Verification items for the finished model (mm, model axes). Give positions to 0.01 mm unless a question says otherwise; leave off trailing zeros. Order: outer loops, then holes, each group sorted by start corner. A loop starts at its lowest first (then second) coordinate and runs counter-clockwise, first axis right, second up.
from build123d import *

# Parameters (mm, degrees)
SKETCH1_R                           = 14.2875
BOSS_EXTRUDE1_DEPTH                 = 6.35
F_0_257_DIAMETER_HOLE1_D            = 6.5278
F_9_0_2_DIAMETER_HOLE1_D            = 5.08
FILLET2_R                           = 12.7
FILLET1_R                           = 19.05
F_9_0_196_DIAMETER_HOLE1_AT_2_COUNT = 2
F_9_0_196_DIAMETER_HOLE1_AT_2_PITCH = 25.4
F_9_0_196_DIAMETER_HOLE1_AT_3_COUNT = 2
F_9_0_196_DIAMETER_HOLE1_AT_3_PITCH = 76.2
F_9_0_196_DIAMETER_HOLE1_AT_4_COUNT = 2
F_9_0_196_DIAMETER_HOLE1_AT_4_PITCH = 101.6


with BuildPart() as part:
    # Sketch1 → Boss-Extrude1 (new body)
    with BuildSketch(Plane.YZ):
        with BuildLine():
            Line((0, -50.8), (-201.989896777, -50.8))
            ThreePointArc((-201.989896777, -50.8), (-204.733971085, -38.269563411), (-206.701492618, -25.593970963))
            Line((-206.701492618, -25.593970963), (-265.489896777, -25.593970963))
            Line((-265.489896777, -25.593970963), (-265.489896777, 50.8))
            Line((-265.489896777, 50.8), (-201.989896777, 50.8))
            Line((-201.989896777, 50.8), (0, 50.8))
            ThreePointArc((0, 50.8), (50.8, 0), (0, -50.8))
        make_face()
        with Locations(Location((0, 0, 0), (0, 0, 270))):
            Circle(SKETCH1_R, mode=Mode.SUBTRACT)
        with Locations(Location((-233.739896777, 12.603014519, 0), (0, 0, 270))):
            Circle(SKETCH1_R, mode=Mode.SUBTRACT)
    extrude(amount=BOSS_EXTRUDE1_DEPTH)

    # F (0.257) Diameter Hole1 (through all)
    with Locations(Plane.YZ.offset(6.35)):
        with Locations((0, 0), (-191.833069099, -38.1), (-195.58, 0), (-191.833069099, 38.1)):
            Hole(F_0_257_DIAMETER_HOLE1_D / 2)

    # #9 (0.2) Diameter Hole1 (through all)
    with Locations(Plane.YZ.offset(6.35)):
        with Locations((-259.139896777, 12.603014519), (-208.339896777, 12.603014519)):
            Hole(F_9_0_2_DIAMETER_HOLE1_D / 2)

    # Fillet2
    fillet2_edges = [part.edges().sort_by_distance(p)[0] for p in [
        (3.175, -265.489896777, -25.593970963),
        (3.175, -265.489896777, 50.8),
    ]]
    fillet(fillet2_edges, radius=FILLET2_R)

    # Fillet1
    fillet1_edges = [part.edges().sort_by_distance(p)[0] for p in [
        (3.175, -206.701492618, -25.593970963),
    ]]
    fillet(fillet1_edges, radius=FILLET1_R)

    # Sketch9 → #9 (0.196) Diameter Hole1 (revolve, cut)
    with BuildSketch(Plane(origin=(6.35, -163.889896777, -38.1), x_dir=(0, 0, -1), z_dir=(0, 1, 0))):
        Polygon((0, 0), (0, 6.35), (4.7625, 6.35), (2.4892, 4.0767), (2.4892, 0), align=None)
    f_9_0_196_diameter_hole1 = revolve(axis=Axis((12.7, -163.889896777, -38.1), (-1, 0, 0)), mode=Mode.SUBTRACT)

    # #9 (0.196) Diameter Hole1 at 2: #9 (0.196) Diameter Hole1 ×2
    with Locations(*[(0, i * F_9_0_196_DIAMETER_HOLE1_AT_2_PITCH, 0) for i in range(1, F_9_0_196_DIAMETER_HOLE1_AT_2_COUNT)]):
        add(f_9_0_196_diameter_hole1, mode=Mode.SUBTRACT)

    # #9 (0.196) Diameter Hole1 at 3: #9 (0.196) Diameter Hole1 ×2
    with Locations(*[(0, i * F_9_0_196_DIAMETER_HOLE1_AT_3_PITCH, 0) for i in range(1, F_9_0_196_DIAMETER_HOLE1_AT_3_COUNT)]):
        add(f_9_0_196_diameter_hole1, mode=Mode.SUBTRACT)

    # #9 (0.196) Diameter Hole1 at 4: #9 (0.196) Diameter Hole1 ×2
    with Locations(*[(0, i * F_9_0_196_DIAMETER_HOLE1_AT_4_PITCH, 0) for i in range(1, F_9_0_196_DIAMETER_HOLE1_AT_4_COUNT)]):
        add(f_9_0_196_diameter_hole1, mode=Mode.SUBTRACT)


solid = part.part
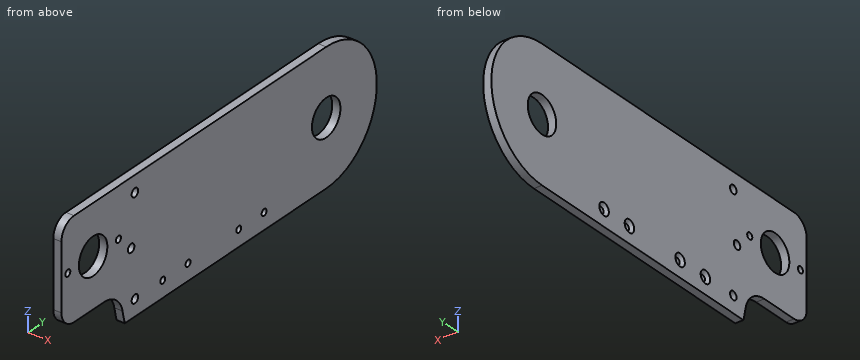
(1) Go/stop test with a flat-tipped pin: pin 1 (3 mm diameter, centred on x = 4, y = -232, fed in from -Z). Record where the tip stops, or that it passes through.
Solved:
pin 1: stops at z = -25.59
(2) Section check A-A, the plane x = 1. Give the number of separate pieces and of enclosed holes in the cut face, then the cut area to 3 significant figures.
Solved:
separate pieces: 1
enclosed holes: 11
area: 27,900 mm2
(3) Section check B-B, the plane z = -28.5. Enter the section's corners in (x, y).
Solved:
outline: (0, -212.79) - (6.35, -212.79) - (6.35, 42.05) - (0, 42.05) - close
(4) Scan lines: line 1 (Y direction, x = 1.5, z = 1); line 2 (Y direction, x = 5, z = 8); line 3 (Y direction, x = 4.5, z = 9). Record each from-to range of solid material in increasing order.
Solved:
line 1: y = -265.49 to -242.08, -225.4 to -198.69, -192.47 to -14.25, 14.25 to 50.79
line 2: y = -265.49 to -247.27, -220.21 to -11.84, 11.84 to 50.17
line 3: y = -265.49 to -247.57, -219.91 to -11.1, 11.1 to 50
